```python
from build123d import *

# Parameters (mm, degrees)
SKETCH_1_R               = 1.75
EXTRUDE_1_DEPTH          = 15
EXTRUDE_1_2_DEPTH        = 15
EXTRUDE_1_3_DEPTH        = 15
EXTRUDE_1_4_DEPTH        = 15
EXTRUDE_1_5_DEPTH        = 15
EXTRUDE_1_6_DEPTH        = 15
EXTRUDE_1_7_DEPTH        = 15
EXTRUDE_1_8_DEPTH        = 15
SKETCH_2_R               = 48.25
EXTRUDE_2_DEPTH          = 5
EXTRUDE_START            = -15
SKETCH_3_R               = 53.25
SKETCH_3_R_2             = 48.25
EXTRUDE_1_9_DEPTH        = 15
SKETCH_4_R               = 60
SKETCH_4_R_2             = 48.25
EXTRUDE_3_DEPTH          = 4
CUT_EXTRUDE_1_REACH      = 87.563
SKETCH_6_R               = 1.5
CUT_EXTRUDE_3_DEPTH      = 94.407708461
CUT_EXTRUDE_3_DEPTH_BACK = 94.407708461
SKETCH_9_W               = 50
SKETCH_9_H               = 10
SKETCH_10_R              = 53.25
EXTRUDE_4_DEPTH          = 5
CUT_EXTRUDE_4_DEPTH      = 89.459030065
CUT_EXTRUDE_4_DEPTH_BACK = 89.459030065
SKETCH_11_R              = 1.75


with BuildPart() as part:
    # Sketch 1 → Extrude 1 (new body)
    with BuildSketch(Plane.XY):
        with Locations((43.431304103, -0.032870953)):
            Circle(SKETCH_1_R)
    extrude(amount=EXTRUDE_1_DEPTH)



with BuildPart() as body_2:
    # Sketch 1 → Extrude 1 2 (new body)
    with BuildSketch(Plane.XY):
        with Locations((31.159786222, -30.557369002)):
            Circle(SKETCH_1_R)
    extrude(amount=EXTRUDE_1_2_DEPTH)


with BuildPart() as body_3:
    # Sketch 1 → Extrude 1 3 (new body)
    with BuildSketch(Plane.XY):
        with Locations((0.89843315, -43.464175056)):
            Circle(SKETCH_1_R)
    extrude(amount=EXTRUDE_1_3_DEPTH)


with BuildPart() as body_4:
    # Sketch 1 → Extrude 1 4 (new body)
    with BuildSketch(Plane.XY):
        with Locations((-29.626064899, -31.192657175)):
            Circle(SKETCH_1_R)
    extrude(amount=EXTRUDE_1_4_DEPTH)


with BuildPart() as body_5:
    # Sketch 1 → Extrude 1 5 (new body)
    with BuildSketch(Plane.XY):
        with Locations((-42.532870953, -0.931304103)):
            Circle(SKETCH_1_R)
    extrude(amount=EXTRUDE_1_5_DEPTH)


with BuildPart() as body_6:
    # Sketch 1 → Extrude 1 6 (new body)
    with BuildSketch(Plane.XY):
        with Locations((-30.261353072, 29.593193946)):
            Circle(SKETCH_1_R)
    extrude(amount=EXTRUDE_1_6_DEPTH)


with BuildPart() as body_7:
    # Sketch 1 → Extrude 1 7 (new body)
    with BuildSketch(Plane.XY):
        with Locations((0, 42.5)):
            Circle(SKETCH_1_R)
    extrude(amount=EXTRUDE_1_7_DEPTH)


with BuildPart() as body_8:
    # Sketch 1 → Extrude 1 8 (new body)
    with BuildSketch(Plane.XY):
        with Locations((30.524498049, 30.228482119)):
            Circle(SKETCH_1_R)
    extrude(amount=EXTRUDE_1_8_DEPTH)


with BuildPart() as part_1:
    add(part.part)

    add(body_2.part)  # Extrude 2 merges body 2

    add(body_3.part)  # Extrude 2 merges body 3

    add(body_4.part)  # Extrude 2 merges body 4

    add(body_5.part)  # Extrude 2 merges body 5

    add(body_6.part)  # Extrude 2 merges body 6

    add(body_7.part)  # Extrude 2 merges body 7

    add(body_8.part)  # Extrude 2 merges body 8
    # Sketch 2 → Extrude 2 (add)
    with BuildSketch(Plane.XY):
        Circle(SKETCH_2_R)
    extrude(amount=-EXTRUDE_2_DEPTH)

    # Sketch 3 → Extrude 1 9 (add)
    with BuildSketch(Plane(origin=(0, 0, -5), x_dir=(-1, 0, 0), z_dir=(0, 0, -1)).offset(EXTRUDE_START)):
        Circle(SKETCH_3_R)
        Circle(SKETCH_3_R_2, mode=Mode.SUBTRACT)
    extrude(amount=EXTRUDE_1_9_DEPTH)

    # Sketch 4 → Extrude 3 (add)
    with BuildSketch(Plane.XY.offset(10)):
        Circle(SKETCH_4_R)
        with Locations(Location((0, 0, 0), (0, 0, 180))):
            Circle(SKETCH_4_R_2, mode=Mode.SUBTRACT)
    extrude(amount=-EXTRUDE_3_DEPTH)

    # Sketch 6 → Cut-Extrude 1 (cut, up to next)
    with BuildSketch(Plane(origin=(0, 0, 6), x_dir=(-1, 0, 0), z_dir=(0, 0, -1)), mode=Mode.PRIVATE) as cut_extrude_1_sk1:
        with Locations((0, 57)):
            Circle(SKETCH_6_R)
    cut_extrude_1_tool1 = extrude(cut_extrude_1_sk1.sketch, amount=-CUT_EXTRUDE_1_REACH, mode=Mode.PRIVATE) & part_1.part
    # Sketch 6 → Cut-Extrude 1 (cut, up to next)
    with BuildSketch(Plane(origin=(0, 0, 6), x_dir=(-1, 0, 0), z_dir=(0, 0, -1)), mode=Mode.PRIVATE) as cut_extrude_1_sk2:
        with Locations((49.363448016, 28.5)):
            Circle(SKETCH_6_R)
    cut_extrude_1_tool2 = extrude(cut_extrude_1_sk2.sketch, amount=-CUT_EXTRUDE_1_REACH, mode=Mode.PRIVATE) & part_1.part
    # Sketch 6 → Cut-Extrude 1 (cut, up to next)
    with BuildSketch(Plane(origin=(0, 0, 6), x_dir=(-1, 0, 0), z_dir=(0, 0, -1)), mode=Mode.PRIVATE) as cut_extrude_1_sk3:
        with Locations((49.363448016, -28.5)):
            Circle(SKETCH_6_R)
    cut_extrude_1_tool3 = extrude(cut_extrude_1_sk3.sketch, amount=-CUT_EXTRUDE_1_REACH, mode=Mode.PRIVATE) & part_1.part
    # Sketch 6 → Cut-Extrude 1 (cut, up to next)
    with BuildSketch(Plane(origin=(0, 0, 6), x_dir=(-1, 0, 0), z_dir=(0, 0, -1)), mode=Mode.PRIVATE) as cut_extrude_1_sk4:
        with Locations((0, -57)):
            Circle(SKETCH_6_R)
    cut_extrude_1_tool4 = extrude(cut_extrude_1_sk4.sketch, amount=-CUT_EXTRUDE_1_REACH, mode=Mode.PRIVATE) & part_1.part
    # Sketch 6 → Cut-Extrude 1 (cut, up to next)
    with BuildSketch(Plane(origin=(0, 0, 6), x_dir=(-1, 0, 0), z_dir=(0, 0, -1)), mode=Mode.PRIVATE) as cut_extrude_1_sk5:
        with Locations((-49.363448016, -28.5)):
            Circle(SKETCH_6_R)
    cut_extrude_1_tool5 = extrude(cut_extrude_1_sk5.sketch, amount=-CUT_EXTRUDE_1_REACH, mode=Mode.PRIVATE) & part_1.part
    # Sketch 6 → Cut-Extrude 1 (cut, up to next)
    with BuildSketch(Plane(origin=(0, 0, 6), x_dir=(-1, 0, 0), z_dir=(0, 0, -1)), mode=Mode.PRIVATE) as cut_extrude_1_sk6:
        with Locations((-49.363448016, 28.5)):
            Circle(SKETCH_6_R)
    cut_extrude_1_tool6 = extrude(cut_extrude_1_sk6.sketch, amount=-CUT_EXTRUDE_1_REACH, mode=Mode.PRIVATE) & part_1.part
    add(cut_extrude_1_tool1.solids().sort_by_distance((0, 57, 6))[0], mode=Mode.SUBTRACT)
    add(cut_extrude_1_tool2.solids().sort_by_distance((-49.363448, 28.5, 6))[0], mode=Mode.SUBTRACT)
    add(cut_extrude_1_tool3.solids().sort_by_distance((-49.363448, -28.5, 6))[0], mode=Mode.SUBTRACT)
    add(cut_extrude_1_tool4.solids().sort_by_distance((0, -57, 6))[0], mode=Mode.SUBTRACT)
    add(cut_extrude_1_tool5.solids().sort_by_distance((49.363448, -28.5, 6))[0], mode=Mode.SUBTRACT)
    add(cut_extrude_1_tool6.solids().sort_by_distance((49.363448, 28.5, 6))[0], mode=Mode.SUBTRACT)

    # Sketch 9 → Cut-Extrude 3 (cut, two sides: drawn at the far end of the back side and taken through both)
    with BuildSketch(Plane(origin=(0, 10, 0), x_dir=(1, 0, 0), z_dir=(0, 1, 0)).offset(-CUT_EXTRUDE_3_DEPTH_BACK)):
        with Locations((0, -1)):
            Rectangle(SKETCH_9_W, SKETCH_9_H)
    extrude(amount=CUT_EXTRUDE_3_DEPTH + CUT_EXTRUDE_3_DEPTH_BACK, mode=Mode.SUBTRACT)


with BuildPart() as body_2_2:
    # of the pieces the cut leaves, the one that is kept (cut_extrude_3_keep)
    add(part_1.part.solids().sort_by_distance((-25, 41.268177813, 0))[0])

    # Sketch 10 → Extrude 4 (add)
    with BuildSketch(Plane(origin=(0, 0, -5), x_dir=(-1, 0, 0), z_dir=(0, 0, -1))):
        Circle(SKETCH_10_R)
    extrude(amount=EXTRUDE_4_DEPTH)

    # Sketch 11 → Cut-Extrude 4 (cut, two sides: drawn at the far end of the back side and taken through both)
    with BuildSketch(Plane(origin=(0, 0, -10), x_dir=(-1, 0, 0), z_dir=(0, 0, -1)).offset(-CUT_EXTRUDE_4_DEPTH_BACK)):
        with Locations((30.261353072, 29.593193946)):
            Circle(SKETCH_11_R)
        with Locations((42.532870953, -0.931304103)):
            Circle(SKETCH_11_R)
        with Locations((29.626064899, -31.192657175)):
            Circle(SKETCH_11_R)
        with Locations((-31.159786222, -30.557369002)):
            Circle(SKETCH_11_R)
        with Locations((-43.431304103, -0.032870953)):
            Circle(SKETCH_11_R)
        with Locations((-30.524498049, 30.228482119)):
            Circle(SKETCH_11_R)
    extrude(amount=CUT_EXTRUDE_4_DEPTH + CUT_EXTRUDE_4_DEPTH_BACK, mode=Mode.SUBTRACT)


solid = body_2_2.part
```
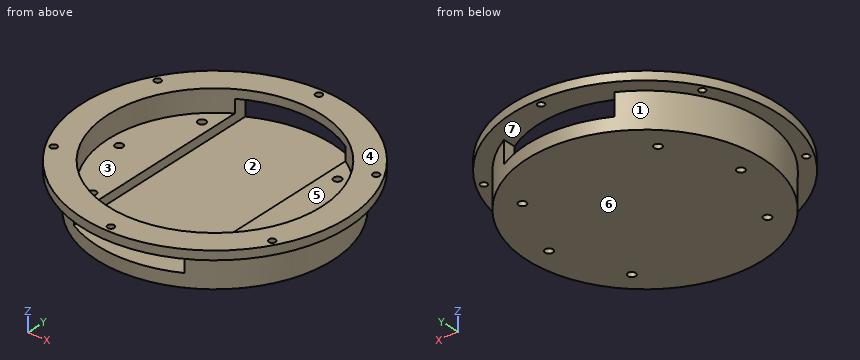
The model under review builds one solid part; all positions refer to its coordinate system, in mm. Face numbers are marked on the shaded views. A direction names the side the tool comes from. Coordinates: 2 decimals unless noted, no trailing zeros. Write each loop counter-clockwise with the first axis right and the second up, starting at its lowest first coordinate (ties: lowest second). Pieces come first, ordered by that corner, then holes. Notation, with made-up numbers: (29, 70.5) - (44, 70.5) arc R34 cw to (44, 105.5) - close; hole circle Ø11 at (84, 14.25). An arc over 180 degrees is marked (long way). Answer in a Markdown table with one row per item. Add a question column.
Q1. Consider section A-A on x = 0. Give the boundary of the cut face in (y, z), then the cut area to 3 significant figures.
Q2. For the marked faces 1, 2, 3 and 4, list the 3-axis set-ups (+Z, -Z, +X, -X, +Y, -Y) from which the entire face can be reached by the end or side of a thin tool; tool diameter is ignored.
Q3. Consider section D-D on x = 20. Give the boundary of the cut face in (y, z), then the cut area to 3 significant figures.
Q4. Clearance check with flat-ended pins moving along their axes: pin 1 (6 mm diameter, centred on x = 41, z = -0.5, fed in from -Y); pin 2 (3 mm diameter, centred on x = -29.5, z = -6, fed in from +Y); pin 3 (3 mm diameter, centred on y = 6, z = 0.5, fed in from -X). State where each tip first meets the part, or that it passes through.
Q5. Draft analysis for pull direction Z (two halves, no side actions). For the marked faces 5, 6 and 7, state which applies: +Z half, -Z half, draft (parallel to the pull), parting line (faces both ways), or undercut.
Q6. Consider section B-B on y = -57. Give the boundary of the cut face in (x, z) (3 decimals).
Q7. To check wall thickness, follow line 1 along Z through (x, y) = (13.5, 6.5); line 2 along Z through (x, y) = (-35, -21); line 3 along X through (y, z) = (32, 2.5). State the ranges of each line that lie inside material, in increasing order. Write a range as from..to.
Q8. Consider section C-C on z = -7.5. Give the boundary of the cut face in (x, y), then the cut area to 3 significant figures.
Answers below:
| question | item | result |
|---|---|---|
| 1 | outline | (-60, 6) - (-58.5, 6) - (-58.5, 10) - (-60, 10) - close; (-55.5, 6) - (-48.25, 6) - (-48.25, 10) - (-55.5, 10) - close; (-53.25, -10) - (53.25, -10) - (53.25, -4) - (-53.25, -4) - close; (48.25, 6) - (55.5, 6) - (55.5, 10) - (48.25, 10) - close; (58.5, 6) - (60, 6) - (60, 10) - (58.5, 10) - close |
| 1 | area | 709 mm² |
| 2 | face 1 | -Z |
| 2 | face 2 | +Y, -Y |
| 2 | face 3 | +Z |
| 2 | face 4 | +Z, +X, -X, +Y, -Y |
| 3 | outline | (-56.57, 6) - (-43.91, 6) - (-43.91, 10) - (-56.57, 10) - close; (-49.35, -10) - (49.35, -10) - (49.35, -4) - (-49.35, -4) - close; (43.91, 6) - (56.57, 6) - (56.57, 10) - (43.91, 10) - close |
| 3 | area | 693 mm² |
| 4 | pin 1 | y = -37.3 |
| 4 | pin 2 | y = 45.29 |
| 4 | pin 3 | x = -53.06 |
| 5 | face 5 | +Z half |
| 5 | face 6 | -Z half |
| 5 | face 7 | undercut |
| 6 | outline | (-18.735, 6) - (-1.5, 6) - (-1.5, 10) - (-18.735, 10) - close; (1.5, 6) - (18.735, 6) - (18.735, 10) - (1.5, 10) - close |
| 7 | line 1 | -10..-4 |
| 7 | line 2 | -10..0 |
| 7 | line 3 | -42.56..-36.11, 36.11..42.56 |
| 8 | outline | circle Ø106.5 at (0, 0); hole circle Ø3.5 at (-42.53, -0.93); hole circle Ø3.5 at (-30.26, 29.59); hole circle Ø3.5 at (-29.63, -31.19); hole circle Ø3.5 at (30.52, 30.23); hole circle Ø3.5 at (31.16, -30.56); hole circle Ø3.5 at (43.43, -0.03) |
| 8 | area | 8,850 mm² |
